Geometry check sheet. Reference: the model listing, model coordinates, mm. Coordinates: 2 decimals unless noted, no trailing zeros. Write each loop counter-clockwise with the first axis right and the second up, starting at its lowest first coordinate (ties: lowest second). Pieces come first, ordered by that corner, then holes. Notation, with made-up numbers: (-36.5, 9.25) -> (18.5, 9.25) arc R23 cw to (18.5, 20.25) -> close; hole circle Ø7 at (28.5, 11.5). An arc over 180 degrees is marked (long way). Answer in a Markdown table with one row per item. Add a question column.
1. Cross-section at C-C on y = 1.15. Give the number of separate pieces and of enclosed holes in the cut face, and give its area (3 significant figures).
2. Cross-section at B-B on z = 8. Record the cut outline in (x, y).
3. Depth check by flat-ended pin: P1, Ø1, axis at y = 0.5, z = 37.5, coming from the +X side; P2, Ø1.5, axis at y = 1, z = 45.5, coming from the -X side; P3, Ø1.5, axis at x = 30, y = 1.5, coming from the +Z side. Enter the tip coordinate at first touch or a pass-through.
4. Cross-section at A-A on x = 35. Record the cut outline in (y, z), and give its area (3 significant figures).
5. Cross-section at D-D on z = 17. Record the cut outline in (x, y).
6. Scan lines: L1, parallel to Z at x = -11, y = 2.95; L2, parallel to Z at x = -9.5, y = 1; L3, parallel to X at y = 0.65, z = -13. Record each from-to range of solid material in increasing order. Write a range as from..to.
```python
from build123d import *

# Parameters (mm, degrees)
SZKIC1_R                   = 2.1
SZKIC1_R_2                 = 12.5
WYCI_GNI_CIE_PROSTE1_DEPTH = 3
ZAOKR_GLENIE1_R            = 0.5
ZAOKR_GLENIE3_R            = 3.5
ZAOKR_GLENIE4_R            = 7
ZAOKR_GLENIE5_R            = 70
ZAOKR_GLENIE6_R            = 49
ZAOKR_GLENIE7_R            = 49
ZAOKR_GLENIE8_R            = 7


with BuildPart() as part:
    # Szkic1 → Wyciągnięcie proste1 (new body)
    with BuildSketch(Plane(origin=(0, 0, 0), x_dir=(-1, 0, 0), z_dir=(0, 1, 0))):
        Polygon((-18.25, -18.25), (18.25, -18.25), (18.25, 18.25), (-5.78812344, 53.629485271), (-35.78812344, 53.629485271), (-45.78812344, 53.629485271), (-45.78812344, 46.129485271), (-25.28812344, 46.129485271), (-25.28812344, 5.129485271), (-45.78812344, 5.129485271), (-45.78812344, -2.870514729), align=None)
        with Locations(Location((-40.78812344, 1.629485271, 0), (0, 0, 270))):
            Circle(SZKIC1_R, mode=Mode.SUBTRACT)
        with Locations(Location((-12.5, 12.5, 0), (0, 0, 270))):
            Circle(SZKIC1_R, mode=Mode.SUBTRACT)
        with Locations(Location((-30.78812344, 49.629485271, 0), (0, 0, 270))):
            Circle(SZKIC1_R, mode=Mode.SUBTRACT)
        with Locations(Location((-40.78812344, 49.629485271, 0), (0, 0, 270))):
            Circle(SZKIC1_R, mode=Mode.SUBTRACT)
        with Locations(Location((12.5, 12.5, 0), (0, 0, 270))):
            Circle(SZKIC1_R, mode=Mode.SUBTRACT)
        with Locations(Location((-30.78812344, 1.629485271, 0), (0, 0, 270))):
            Circle(SZKIC1_R, mode=Mode.SUBTRACT)
        with Locations(Location((12.5, -12.5, 0), (0, 0, 270))):
            Circle(SZKIC1_R, mode=Mode.SUBTRACT)
        with Locations(Location((-12.5, -12.5, 0), (0, 0, 270))):
            Circle(SZKIC1_R, mode=Mode.SUBTRACT)
        with Locations(Location((0, 0, 0), (0, 0, 270))):
            Circle(SZKIC1_R_2, mode=Mode.SUBTRACT)
    extrude(amount=WYCI_GNI_CIE_PROSTE1_DEPTH)

    # Zaokrąglenie1
    zaokr_glenie1_edges = [part.edges().sort_by_distance(p)[0] for p in [
        (25.28812344, 1.5, 5.129485271),
        (25.28812344, 1.5, 46.129485271),
    ]]
    fillet(zaokr_glenie1_edges, radius=ZAOKR_GLENIE1_R)

    # Zaokrąglenie3
    zaokr_glenie3_edges = [part.edges().sort_by_distance(p)[0] for p in [
        (45.78812344, 1.5, 5.129485271),
        (45.78812344, 1.5, 46.129485271),
        (45.78812344, 1.5, 53.629485271),
    ]]
    fillet(zaokr_glenie3_edges, radius=ZAOKR_GLENIE3_R)

    # Zaokrąglenie4
    zaokr_glenie4_edges = [part.edges().sort_by_distance(p)[0] for p in [
        (45.78812344, 1.5, -2.870514729),
    ]]
    fillet(zaokr_glenie4_edges, radius=ZAOKR_GLENIE4_R)

    # Zaokrąglenie5
    zaokr_glenie5_edges = [part.edges().sort_by_distance(p)[0] for p in [
        (18.25, 1.5, -18.25),
    ]]
    fillet(zaokr_glenie5_edges, radius=ZAOKR_GLENIE5_R)

    # Zaokrąglenie6
    zaokr_glenie6_edges = [part.edges().sort_by_distance(p)[0] for p in [
        (5.78812344, 1.5, 53.629485271),
    ]]
    fillet(zaokr_glenie6_edges, radius=ZAOKR_GLENIE6_R)

    # Zaokrąglenie7
    zaokr_glenie7_edges = [part.edges().sort_by_distance(p)[0] for p in [
        (-18.25, 1.5, 18.25),
    ]]
    fillet(zaokr_glenie7_edges, radius=ZAOKR_GLENIE7_R)

    # Zaokrąglenie8
    zaokr_glenie8_edges = [part.edges().sort_by_distance(p)[0] for p in [
        (-18.25, 1.5, -18.25),
    ]]
    fillet(zaokr_glenie8_edges, radius=ZAOKR_GLENIE8_R)


solid = part.part
```
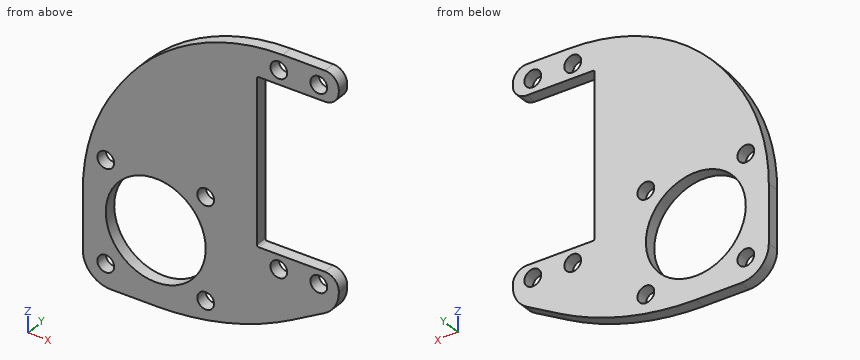
Results found:
| question | item | result |
|---|---|---|
| 1 | separate pieces | 1 |
| 1 | enclosed holes | 9 |
| 1 | area | 2,350 mm^2 |
| 2 | outline | (-18.01, 0) -> (-9.6, 0) -> (-9.6, 3) -> (-18.01, 3) -> close; (9.6, 0) -> (25.29, 0) -> (25.29, 3) -> (9.6, 3) -> close |
| 3 | P1 | stops at x = 25.29 |
| 3 | P2 | stops at x = 3.6 |
| 3 | P3 | stops at z = 53.62 |
| 4 | outline | (0, -8.9) -> (3, -8.9) -> (3, 5.13) -> (0, 5.13) -> close; (0, 46.13) -> (3, 46.13) -> (3, 53.63) -> (0, 53.63) -> close |
| 4 | area | 64.6 mm^2 |
| 5 | outline | (-16.26, 0) -> (25.29, 0) -> (25.29, 3) -> (-16.26, 3) -> close |
| 6 | L1 | z = -18.25..-13.97, -11.03..-5.94, 5.94..11.03, 13.97..28.83 |
| 6 | L2 | z = -18.25..-8.12, 8.12..31.13 |
| 6 | L3 | x = -18.03..-14.54, -10.46..10.46, 14.54..26.63 |
